from build123d import *

# Parameters (mm, degrees)
SKETCH1_R           = 1.5
SKETCH1_R_2         = 1
SKETCH1_R_3         = 7
SKETCH1_R_4         = 4.75
BOSS_EXTRUDE1_DEPTH = 3
BOSS_EXTRUDE2_DEPTH = 8
SKETCH4_R           = 6.5
CUT_EXTRUDE1_DEPTH  = 10


with BuildPart() as part:
    # Sketch1 → Boss-Extrude1 (new body)
    with BuildSketch(Plane(origin=(0, 0, 0), x_dir=(0, 0, -1), z_dir=(1, 0, 0))):
        with BuildLine():
            Line((-49.159345461, 0), (49.159345461, 0))
            ThreePointArc((49.159345461, 0), (66.340654539, 11.242329364), (62.91845049, 31.487720707))
            ThreePointArc((62.91845049, 31.487720707), (56.432557087, 41.829379484), (54.166473214, 53.824444444))
            Line((54.166473214, 53.824444444), (41.340654539, 60.8))
            ThreePointArc((41.340654539, 60.8), (16.928001378, 53.587346839), (9.715348216, 78))
            Line((9.715348216, 78), (-3.110470459, 84.975555556))
            Line((-3.110470459, 84.975555556), (-4.066026015, 83.218594093))
            ThreePointArc((-4.066026015, 83.218594093), (-51.126972403, 116.596460909), (-104.705915866, 138))
            ThreePointArc((-104.705915866, 138), (-115.275757126, 127.38864025), (-105.87300769, 115.730561375))
            ThreePointArc((-105.87300769, 115.730561375), (-51.706077225, 91.471635272), (-16.759345461, 43.5))
            ThreePointArc((-16.759345461, 43.5), (-21.006297134, 33.246951673), (-31.259345461, 29))
            Line((-31.259345461, 29), (-49.159345461, 29))
            ThreePointArc((-49.159345461, 29), (-63.659345461, 14.5), (-49.159345461, 0))
        make_face()
        with Locations((58.840654539, 11.242329364)):
            Circle(SKETCH1_R, mode=Mode.SUBTRACT)
        with Locations((53.840654539, 21.242329364)):
            Circle(SKETCH1_R_2, mode=Mode.SUBTRACT)
        with Locations((-48.659345461, 14.5)):
            Circle(SKETCH1_R_3, mode=Mode.SUBTRACT)
        with Locations((-105.289461778, 126.865280687)):
            Circle(SKETCH1_R_4, mode=Mode.SUBTRACT)
        with BuildLine():
            Line((45.840654539, 15.742329364), (47.840654539, 15.742329364))
            ThreePointArc((47.840654539, 15.742329364), (52.340654539, 11.242329364), (47.840654539, 6.742329364))
            Line((47.840654539, 6.742329364), (45.840654539, 6.742329364))
            ThreePointArc((45.840654539, 6.742329364), (41.340654539, 11.242329364), (45.840654539, 15.742329364))
        make_face(mode=Mode.SUBTRACT)
        with BuildLine():
            Line((-86.096000708, 120.210043762), (-79.987998673, 117.98691283))
            ThreePointArc((-79.987998673, 117.98691283), (-78.643235599, 115.103059111), (-81.527089318, 113.758296037))
            Line((-81.527089318, 113.758296037), (-87.635091353, 115.981426968))
            ThreePointArc((-87.635091353, 115.981426968), (-88.979854428, 118.865280687), (-86.096000708, 120.210043762))
        make_face(mode=Mode.SUBTRACT)
        with BuildLine():
            Line((-77.104144954, 124.438660555), (-70.996142919, 122.215529624))
            ThreePointArc((-70.996142919, 122.215529624), (-69.651379845, 119.331675904), (-72.535233564, 117.98691283))
            Line((-72.535233564, 117.98691283), (-78.643235599, 120.210043762))
            ThreePointArc((-78.643235599, 120.210043762), (-79.987998673, 123.093897481), (-77.104144954, 124.438660555))
        make_face(mode=Mode.SUBTRACT)
    extrude(amount=BOSS_EXTRUDE1_DEPTH)

    # Sketch2 → Boss-Extrude2 (add)
    with BuildSketch(Plane(origin=(3, 0, 0), x_dir=(0, 0, -1), z_dir=(1, 0, 0))):
        Polygon((43.976096732, 59.366666667), (51.003942582, 55.544444444), (43.837275915, 42.367233477), (36.809430066, 46.189455699), align=None)
        Polygon((-0.650724412, 83.637777778), (6.377121438, 79.815555556), (-0.789545229, 66.638344588), (-7.817391078, 70.46056681), align=None)
    extrude(amount=BOSS_EXTRUDE2_DEPTH)

    # Sketch4 → Cut-Extrude1 (cut)
    with BuildSketch(Plane(origin=(3, 0, 0), x_dir=(0, 0, -1), z_dir=(1, 0, 0))):
        with Locations((47.840654539, 11.242329364)):
            Circle(SKETCH4_R)
    extrude(amount=-CUT_EXTRUDE1_DEPTH, mode=Mode.SUBTRACT)


solid = part.part
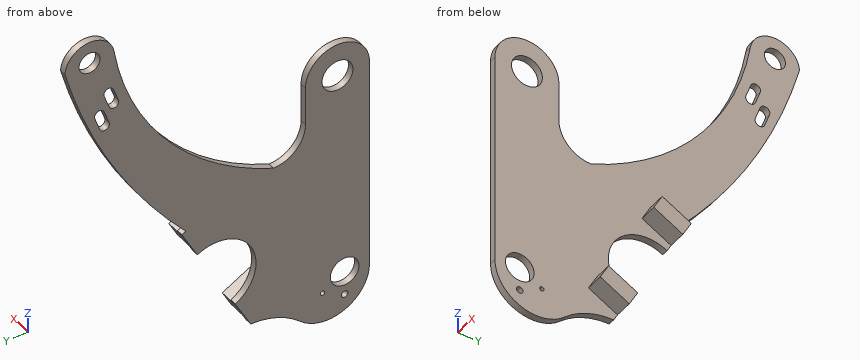
Here's how the part is built. I have some questions about the finished solid (model axes, mm). Round coordinates to 2 decimals unless told otherwise and drop trailing zeros. Write each loop counter-clockwise with the first axis right and the second up, starting at its lowest first coordinate (ties: lowest second). Pieces come first, ordered by that corner, then holes.
1. Suppose I cut it at B-B (y = 40.5). List the corners of the cut face in (x, z) for me, and give its area (3 significant figures).
2. I need wall thicknesses on L1, parallel to X at y = 101, z = 58; L2, parallel to Y at x = 2.25, z = -46.5; L3, parallel to Y at x = 2, z = 51. Which ranges of each line are inside material? Lowest first, please.
3. Will these pins go through, and if not, where does the flat tip stop? pin 1 Ø6 at (x, y) = (3, 98) entering from -Z; pin 2 Ø2.5 at (x, z) = (2, 36.5) entering from +Y; pin 3 Ø1.8 at (y, z) = (11.24, -58.84) entering from +X; pin 4 Ø4 at (x, y) = (3, 103.5) entering from +Z.
4. Suppose I cut it at C-C (y = 26.5). List the corners of the cut face in (x, z) for me.
5. Suppose I cut it at A-A (x = 5). List the corners of the cut face in (y, z) for me, and give its area (3 significant figures).
Answer sheet:
1. outline: (0, -56.99) - (3, -56.99) - (3, 17.07) - (0, 17.07) - close
1. area: 222 mm2
2. L1: x = 0 to 3
2. L2: y = 0 to 4.88, 17.6 to 57.99
2. L3: y = 0.12 to 7.9, 21.1 to 28.88, 90.89 to 116.53
3. pin 1: stops at z = 18.12
3. pin 2: stops at y = 108.75
3. pin 3: passes through
3. pin 4: stops at z = 73.69
4. outline: (0, -66.23) - (3, -66.23) - (3, 57.3) - (0, 57.3) - close
5. outline: (42.37, -43.84) - (55.54, -51) - (59.37, -43.98) - (46.19, -36.81) - close; (66.64, 0.79) - (79.82, -6.38) - (83.64, 0.65) - (70.46, 7.82) - close
5. area: 240 mm2
